Geometry: final body of the model. Coordinates: model frame, mm. Face numbers are marked on the shaded views. Give positions to 0.01 mm unless a question says otherwise; leave off trailing zeros. Write each loop counter-clockwise with the first axis right and the second up, starting at its lowest first coordinate (ties: lowest second). Pieces come first, ordered by that corner, then holes. Notation, with made-up numbers: (89, 88.25) -> (112, 88.25) arc R15 cw to (112, 102.25) -> close; hole circle Ø11 at (62.5, 24). An arc over 180 degrees is marked (long way). Use CSV: the item, a comma, the result in double quotes. Start each with the question number.
1) Section B-B (z = -12). Output: boundary loops of the cut face in (x, y), plus the area to 3 significant figures.
2) Section D-D (z = 1.25). Output: boundary loops of the cut face in (x, y), plus the area to 3 significant figures.
3) Section C-C (y = -2). Output: boundary loops of the cut face in (x, z).
4) Material intervals for line 1 (Z direction, x = 0, y = 1.85); line 2 (Z direction, x = 0, y = 0.9); line 3 (X direction, y = 1.05, z = -20), sorted ascending. Write a range as [from, to].
5) Contact query for flat-ended pins moving along their axis: P1, Ø4, axis at x = -1.5, y = -3, coming from the -Z side; P2, Ø3.5, axis at x = 0, z = 0, coming from the -Y side; P3, Ø2.5, axis at x = 0, z = -16, coming from the +Y side (1 decimal); P4, Ø1.5, axis at y = -2, z = -0.5, coming from the -X side. Output: stop coordinate, or through.
6) Section A-A (x = 0). Count the separate pieces of the cut face and the enclosed holes in it, plus the area to 3 significant figures.
7) Draft query along X for the marked faces 1, 2, 3 and 4. Return one class per face: pulls with the +X half, pulls with the -X half, needs draft (parallel to the pull), parting line crosses it, or undercut.
```python
from build123d import *

# Parameters (mm, degrees)
BOSS_EXTRUDE1_DEPTH = 2
SKETCH2_R           = 1.5
CUT_EXTRUDE1_DEPTH  = 3
SKETCH7_R           = 4.75
BOSS_EXTRUDE2_DEPTH = 5
SKETCH3_R           = 1.5
CUT_EXTRUDE2_DEPTH  = 8
SKETCH4_R           = 3
CUT_EXTRUDE3_DEPTH  = 1.016
SKETCH6_R           = 1.5
CUT_EXTRUDE4_DEPTH  = 8
SKETCH5_R           = 1.5
CUT_EXTRUDE5_DEPTH  = 8
SKETCH8_R           = 3
CUT_EXTRUDE6_DEPTH  = 5


with BuildPart() as part:
    # Sketch1 → Boss-Extrude1 (new body)
    with BuildSketch(Plane(origin=(0, 0, 0), x_dir=(1, 0, 0), z_dir=(0, 1, 0))):
        with BuildLine():
            Line((3.5, 20), (5, 0))
            ThreePointArc((5, 0), (0, -5), (-5, 0))
            Line((-5, 0), (-3.5, 20))
            ThreePointArc((-3.5, 20), (0, 23.5), (3.5, 20))
        make_face()
    extrude(amount=BOSS_EXTRUDE1_DEPTH)

    # Sketch2 → Cut-Extrude1 (cut, through all)
    with BuildSketch(Plane(origin=(0, 2, 0), x_dir=(1, 0, 0), z_dir=(0, 1, 0))):
        with Locations((0, 20)):
            Circle(SKETCH2_R)
    extrude(amount=-CUT_EXTRUDE1_DEPTH, mode=Mode.SUBTRACT)

    # Sketch7 → Boss-Extrude2 (add)
    with BuildSketch(Plane(origin=(0, 0, 0), x_dir=(-1, 0, 0), z_dir=(0, -1, 0))):
        Circle(SKETCH7_R)
    extrude(amount=BOSS_EXTRUDE2_DEPTH)

    # Sketch3 → Cut-Extrude2 (cut, through all)
    with BuildSketch(Plane(origin=(0, 2, 0), x_dir=(1, 0, 0), z_dir=(0, 1, 0))):
        Circle(SKETCH3_R)
    extrude(amount=-CUT_EXTRUDE2_DEPTH, mode=Mode.SUBTRACT)

    # Sketch4 → Cut-Extrude3 (cut)
    with BuildSketch(Plane(origin=(0, 2, 0), x_dir=(1, 0, 0), z_dir=(0, 1, 0))):
        Circle(SKETCH4_R)
    extrude(amount=-CUT_EXTRUDE3_DEPTH, mode=Mode.SUBTRACT)

    # Sketch6 → Cut-Extrude4 (cut, through all)
    with BuildSketch(Plane(origin=(0, 2, 0), x_dir=(1, 0, 0), z_dir=(0, 1, 0))):
        with Locations((0, 16)):
            Circle(SKETCH6_R)
    extrude(amount=-CUT_EXTRUDE4_DEPTH, mode=Mode.SUBTRACT)

    # Sketch5 → Cut-Extrude5 (cut, through all)
    with BuildSketch(Plane(origin=(0, 2, 0), x_dir=(1, 0, 0), z_dir=(0, 1, 0))):
        with Locations((0, 12)):
            Circle(SKETCH5_R)
    extrude(amount=-CUT_EXTRUDE5_DEPTH, mode=Mode.SUBTRACT)

    # Sketch8 → Cut-Extrude6 (cut)
    with BuildSketch(Plane(origin=(0, -5, 0), x_dir=(-1, 0, 0), z_dir=(0, -1, 0))):
        Circle(SKETCH8_R)
    extrude(amount=-CUT_EXTRUDE6_DEPTH, mode=Mode.SUBTRACT)


solid = part.part
```
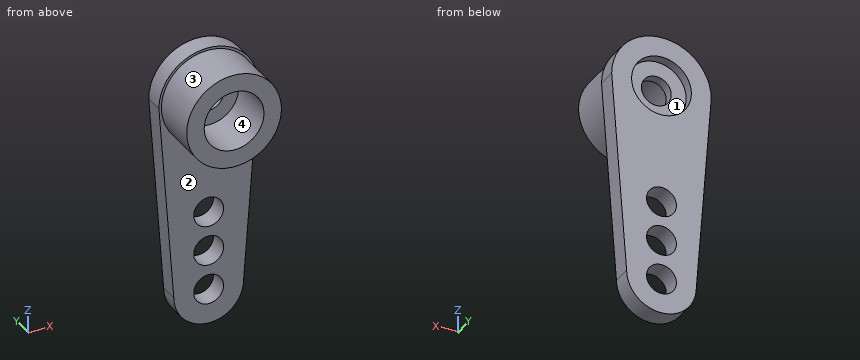
Answers follow:
1,outline,"(-4.1, 0) -> (-1.5, 0) -> (-1.5, 2) -> (-4.1, 2) -> close; (1.5, 0) -> (4.1, 0) -> (4.1, 2) -> (1.5, 2) -> close"
1,area,"10.4 mm^2"
2,outline,"(-4.84, 0) -> (-4.58, 0) -> (-4.58, -5) -> (-2.73, -5) -> (-2.73, 0) -> (-0.83, 0) -> (-0.83, 0.98) -> (-2.73, 0.98) -> (-2.73, 2) -> (-4.84, 2) -> close; (0.83, 0) -> (2.73, 0) -> (2.73, -5) -> (4.58, -5) -> (4.58, 0) -> (4.84, 0) -> (4.84, 2) -> (2.73, 2) -> (2.73, 0.98) -> (0.83, 0.98) -> close"
2,area,"30.7 mm^2"
3,outline,"circle Ø9.5 at (0, 0); hole circle Ø6 at (0, 0)"
4,line 1,"z = [-23.5, -21.5], [-18.5, -17.5], [-14.5, -13.5], [-10.5, -3], [3, 5]"
4,line 2,"z = [-23.5, -21.5], [-18.5, -17.5], [-14.5, -13.5], [-10.5, -1.5], [1.5, 5]"
4,line 3,"x = [-3.5, -1.5], [1.5, 3.5]"
5,P1,"stops at z = -4.75"
5,P2,"stops at y = 0"
5,P3,"passes through"
5,P4,"stops at x = -4.75"
6,separate pieces,"5"
6,enclosed holes,"0"
6,area,"47.5 mm^2"
7,face 1,"undercut"
7,face 2,"needs draft"
7,face 3,"parting line crosses it"
7,face 4,"undercut"
